from build123d import *

# Parameters (mm, degrees)
SKETCH_1_R      = 5.03
SKETCH_1_R_2    = 2
SKETCH_1_R_3    = 9.53
EXTRUDE_1_DEPTH = 4


with BuildPart() as part:
    # 草图1 → 凸台-拉伸1 (new body)
    with BuildSketch(Plane.XY):
        with BuildLine():
            Line((-392.783462019, 31.805361375), (-44.003979129, 80.823121027))
            ThreePointArc((-44.003979129, 80.823121027), (-36.044136208, 80.336276178), (-28.907287603, 76.777974725))
            Line((-28.907287603, 76.777974725), (54.23492213, 11.820161304))
            ThreePointArc((54.23492213, 11.820161304), (59.382296023, -4.260230171), (46.307336141, -14.942920471))
            Line((46.307336141, -14.942920471), (34.224861841, -16))
            Line((34.224861841, -16), (-338.018022509, -16))
            ThreePointArc((-338.018022509, -16), (-341.438223942, -16.603073792), (-344.445898606, -18.339555569))
            Line((-344.445898606, -18.339555569), (-347.211826246, -20.660444431))
            ThreePointArc((-347.211826246, -20.660444431), (-350.219500909, -22.396926208), (-353.639702343, -23))
            Line((-353.639702343, -23), (-390, -23))
            ThreePointArc((-390, -23), (-404.142135624, -17.142135624), (-410, -3))
            Line((-410, -3), (-410, 12))
            ThreePointArc((-410, 12), (-405.094191604, 25.12118058), (-392.783462019, 31.805361375))
        make_face()
        with Locations((45, 0)):
            Circle(SKETCH_1_R, mode=Mode.SUBTRACT)
        with Locations((-55, -11)):
            Circle(SKETCH_1_R_2, mode=Mode.SUBTRACT)
        with Locations((-144.229116997, 61)):
            Circle(SKETCH_1_R_2, mode=Mode.SUBTRACT)
        Circle(SKETCH_1_R_3, mode=Mode.SUBTRACT)
        with Locations((-255, -11)):
            Circle(SKETCH_1_R_2, mode=Mode.SUBTRACT)
        with Locations((-390, 0)):
            Circle(SKETCH_1_R_3, mode=Mode.SUBTRACT)
        with Locations((-35, 74)):
            Circle(SKETCH_1_R_2, mode=Mode.SUBTRACT)
        with Locations((-355, -18)):
            Circle(SKETCH_1_R_2, mode=Mode.SUBTRACT)
        with Locations((-155, -11)):
            Circle(SKETCH_1_R_2, mode=Mode.SUBTRACT)
        with BuildLine():
            Line((-134.303144229, 6), (-50, 6))
            ThreePointArc((-50, 6), (-28.029515257, 29.13921032), (-52.275363905, 49.882018168))
            Line((-52.275363905, 49.882018168), (-127.840019308, 42.024557851))
            ThreePointArc((-127.840019308, 42.024557851), (-132.608278027, 40.222559427), (-135.868840858, 36.304368574))
            Line((-135.868840858, 36.304368574), (-143.366222099, 20.226182617))
            ThreePointArc((-143.366222099, 20.226182617), (-142.737058687, 10.627003917), (-134.303144229, 6))
        make_face(mode=Mode.SUBTRACT)
        with BuildLine():
            Line((-320, 6), (-169.611237636, 6))
            ThreePointArc((-169.611237636, 6), (-164.238241552, 7.566085542), (-160.548159765, 11.773817383))
            Line((-160.548159765, 11.773817383), (-154.850047639, 23.993458271))
            ThreePointArc((-154.850047639, 23.993458271), (-155.76875204, 34.022155928), (-164.94738183, 38.166012783))
            Line((-164.94738183, 38.166012783), (-320.827405056, 21.957097516))
            ThreePointArc((-320.827405056, 21.957097516), (-327.989267179, 13.585741702), (-320, 6))
        make_face(mode=Mode.SUBTRACT)
    extrude(amount=EXTRUDE_1_DEPTH)


solid = part.part
Could you check a few things on this model? Use its own coordinates, in mm. A direction names the side the tool comes from. Round coordinates to 2 decimals unless told otherwise and drop trailing zeros. Loops run counter-clockwise (first coordinate to the right, second up) from the corner with the lowest first, then second, coordinate; pieces in that order, holes last. Notation, with made-up numbers: (45.25, 52) - (86.25, 52) arc R13 ccw to (86.25, 75) - close; hole circle Ø8 at (-6, 71). An arc over 180 degrees is marked (long way). Write item = value, one per line.
1) On a 3-axis mill with a long thin cutter (end or side, diameter ignored), from which of +Z, -Z, +X, -X, +Y, -Y can I reach the whole of each face in a straight line? I mean faces 4 (the flat face through (-139.565, 28.378, 1.972)), 5 (the flat face through (-220.84, 55.97, 1.97)). Say none if no direction works.
Computed:
face_4 = +Z, -Z
face_5 = +Z, -Z, -X, +Y
2) I need wall thicknesses on line 1 along X through (y, z) = (20, 1.65); line 2 along Y through (x, z) = (-55, 1.15); line 3 along Y through (x, z) = (-47.5, 3.5). Which ranges of each line are inside material? Lowest first, please. Write a range as from..to.
Computed:
line_1 = -408.33..-325.29, -156.71..-143.47, -29.51..43.77
line_2 = -16..-13, -9..6, 49.6..79.28
line_3 = -16..6.14, 49.86..80.33
3) If we mould it in two halves opening along X, with no side actions, what happens to faces 1 (the flat face through (-172, 41, 0)), 2 (the cylindrical face through (59.45, -4.02, 1.97)), 3 (the cylindrical face through (-28.01, 28.64, 1.97))? For each: pulls with the +X half, pulls with the -X half, needs draft (parallel to the pull), parting line crosses it, or undercut.
Computed:
face_1 = needs draft
face_2 = pulls with the +X half
face_3 = undercut
4) Imagine slicing it at C-C (x = -122.5). Please give me the cut outline in (y, z), and give its area (3 significant figures).
Computed:
outline = (-16, 0) - (6, 0) - (6, 4) - (-16, 4) - close; (42.58, 0) - (69.79, 0) - (69.79, 4) - (42.58, 4) - close
area = 197 mm2
5) Imagine slicing it at B-B (z = 2.3). Give the number of separate pieces and of enclosed holes in the cut face, and give its area (3 significant figures).
Computed:
separate_pieces = 1
enclosed_holes = 11
area = 23,700 mm2
6) I'm going to push flat-ended pins straight in: P1, Ø2, axis at x = -223, z = 1.5, coming from the +Y side; P2, Ø1, axis at x = -146, z = 1, coming from the +Y side; P3, Ø1.2, axis at x = -80, z = 2, coming from the +Y side; P4, Ø3.5, axis at x = -155, y = -11, coming from the -Z side. Where does each tip first touch, or does it pass through?
Computed:
P1 = 55.81
P2 = 66.56
P3 = 75.85
P4 = through
7) Imagine slicing it at D-D (x = -362). Please give me the cut outline in (y, z), and give its area (3 significant figures).
Computed:
outline = (-23, 0) - (36.13, 0) - (36.13, 4) - (-23, 4) - close
area = 237 mm2
8) Imagine slicing it at A-A (x = -241.5). Please give me the cut outline in (y, z).
Computed:
outline = (-16, 0) - (6, 0) - (6, 4) - (-16, 4) - close; (30.21, 0) - (53.07, 0) - (53.07, 4) - (30.21, 4) - close
